Read the model definition and answer for the solid it produces. Units are mm, in the model's axes. A direction names the side the tool comes from. Coordinates: 2 decimals unless noted, no trailing zeros. Loops run counter-clockwise (first coordinate to the right, second up) from the corner with the lowest first, then second, coordinate; pieces in that order, holes last. Notation, with made-up numbers: (-14, -15.5) -> (-5, -15.5) arc R21 cw to (-5, 9.5) -> close; hole circle Ø10 at (36, 20.25). An arc over 180 degrees is marked (long way). Answer in a Markdown table with one row per item.
```python
from build123d import *

# Parameters (mm, degrees)
F0_R     = 3.175
F1_DEPTH = 3.048


with BuildPart() as f1:
    # F0 (on Top) → F1 (new body)
    with BuildSketch(Plane.XY):
        with BuildLine():
            ThreePointArc((9.525, 114.3), (0.14395, 123.823912), (-9.520649, 114.587868))
            ThreePointArc((-9.520649, 114.587868), (-0.535581, 104.79007), (9.492768, 113.517068))
            ThreePointArc((9.492768, 113.517068), (9.516939, 113.908203), (9.525, 114.3))
        make_face()
        with Locations((0, 114.3)):
            Circle(F0_R, mode=Mode.SUBTRACT)
        with BuildLine():
            Line((-9.520649, 114.587868), (-15.713958, 65.755468))
            ThreePointArc((-15.713958, 65.755468), (-0.703254, 79.359415), (15.452647, 67.137488))
            Line((15.452647, 67.137488), (9.492768, 113.517068))
            ThreePointArc((9.492768, 113.517068), (-0.535581, 104.79007), (-9.520649, 114.587868))
        make_face()
        with Locations((-3.175, 100.0252)):
            Circle(F0_R, mode=Mode.SUBTRACT)
        with BuildLine():
            Line((-15.779489, 65.238779), (-15.779489, 61.761221))
            ThreePointArc((-15.779489, 61.761221), (-1.781346, 47.72526), (14.994367, 58.286115))
            ThreePointArc((14.994367, 58.286115), (15.653293, 60.856134), (15.875, 63.5))
            ThreePointArc((15.875, 63.5), (15.769058, 65.330963), (15.452647, 67.137488))
            ThreePointArc((15.452647, 67.137488), (-0.703254, 79.359415), (-15.713958, 65.755468))
            Line((-15.713958, 65.755468), (-15.779489, 65.238779))
        make_face()
        with Locations((0, 63.5)):
            Circle(F0_R, mode=Mode.SUBTRACT)
        with BuildLine():
            ThreePointArc((-9.23214, 2.343762), (1.180994, 9.451501), (9.525, 0))
            ThreePointArc((9.525, 0), (6.970557, -6.491299), (0.677344, -9.500886))
            Line((0.677344, -9.500886), (44.732405, -7.932475))
            ThreePointArc((44.732405, -7.932475), (36.51336, -0.116834), (44.498789, 7.93735))
            Line((44.498789, 7.93735), (18.996134, 8.094108))
            ThreePointArc((18.996134, 8.094108), (13.152067, 10.707585), (11.129055, 16.781365))
            Line((11.129055, 16.781365), (14.994367, 58.286115))
            ThreePointArc((14.994367, 58.286115), (-1.781346, 47.72526), (-15.779489, 61.761221))
            Line((-15.779489, 61.761221), (-9.23214, 2.343762))
        make_face()
        with BuildLine():
            ThreePointArc((0.677344, -9.500886), (6.970557, -6.491299), (9.525, 0))
            ThreePointArc((9.525, 0), (1.180994, 9.451501), (-9.23214, 2.343762))
            ThreePointArc((-9.23214, 2.343762), (-7.51831, -5.848132), (0, -9.525))
            Line((0, -9.525), (0.677344, -9.500886))
        make_face()
        Circle(F0_R, mode=Mode.SUBTRACT)
        with BuildLine():
            ThreePointArc((44.498789, 7.93735), (36.51336, -0.116834), (44.732405, -7.932475))
            ThreePointArc((44.732405, -7.932475), (50.161633, -5.51191), (52.3875, 0))
            ThreePointArc((52.3875, 0), (50.079883, 5.595384), (44.498789, 7.93735))
        make_face()
        with Locations((44.45, 0)):
            Circle(F0_R, mode=Mode.SUBTRACT)
    extrude(amount=F1_DEPTH)


solid = f1.part
```
1. A cutting plane is placed at C-C on y = 75.5. Give the vertices of the cut face in (x, z).
A:
| item | result |
|---|---|
| outline | (-14.48, 0) -> (14.38, 0) -> (14.38, 3.05) -> (-14.48, 3.05) -> close |
2. A tool of negligible diameter and unlimited length cuts with its end or side. For faces 1 (the cylindrical face through (15.77, 65.31, 1.5)), 2 (the flat face through (13.035, 37.243, 1.503)), from which of +Z, -Z, +X, -X, +Y, -Y can it reach the whole face along a straight path? Write none if from no direction.
A:
| item | result |
|---|---|
| face 1 | +Z, -Z, +X, +Y |
| face 2 | +Z, -Z, +X |
3. Given pin 1 Ø5 at (x, y) = (-3.18, 100.03) entering from -Z; pin 2 Ø1 at (x, z) = (3, 1.5) entering from +Y; pin 3 Ø1 at (x, z) = (20, 0.5) entering from -Y, each flat-ended and moving along its own axis, determine where each tip first touches the part or whether it passes through.
A:
| item | result |
|---|---|
| pin 1 | passes through |
| pin 2 | stops at y = 123.49 |
| pin 3 | stops at y = -8.83 |
4. A cutting plane is placed at A-A on z = 2.45. Count the separate pieces of the cut face and the enclosed holes in it, and give its area (3 significant figures).
A:
| item | result |
|---|---|
| separate pieces | 1 |
| enclosed holes | 5 |
| area | 3,720 mm2 |
5. Find the intervals of material crossed by probe 1 along Y at (x, z) = (44.45, 1.1) (3 decimals); probe 2 along Y at (x, z) = (43, 2.5); probe 3 along Y at (x, z) = (-1.5, 0.7), in increasing order.
A:
| item | result |
|---|---|
| probe 1 | y = -7.943 to -3.175, 3.175 to 7.938 |
| probe 2 | y = -7.99 to -2.82, 2.82 to 7.95 |
| probe 3 | y = -9.41 to -2.8, 2.8 to 60.7, 66.3 to 97.33, 102.72 to 111.5, 117.1 to 123.71 |
6. The mould has two halves that part along X. Classify faces 3 (the cylindrical face through (-0.69, 111.2, 1.5)), 4 (the cylindrical face through (15.647, 60.819, 1.503)), 5 (the cylindrical face through (0.35, 123.82, 1.5)), 6 (the cylindrical face through (-3.588, 103.173, 1.503)): pulls with the +X half, pulls with the -X half, needs draft (parallel to the pull), parting line crosses it, or undercut.
A:
| item | result |
|---|---|
| face 3 | undercut |
| face 4 | pulls with the +X half |
| face 5 | parting line crosses it |
| face 6 | undercut |
7. A cutting plane is placed at B-B on x = 37. Give the vertices of the cut face in (y, z).
A:
| item | result |
|---|---|
| outline | (-8.21, 0) -> (7.98, 0) -> (7.98, 3.05) -> (-8.21, 3.05) -> close |
